Check sheet for the drawn part. Datum: minimum x, y, z corner. Units: mm. Round coordinates to 2 decimals unless told otherwise and drop trailing zeros. Write each loop counter-clockwise with the first axis right and the second up, starting at its lowest first coordinate (ties: lowest second). Pieces come first, ordered by that corner, then holes. Notation, with made-up numbers: (-7, -12) - (31, -12) arc R11 ccw to (31, 8) - close; hole circle Ø5 at (13, -37.5). An arc over 180 degrees is marked (long way). Return JSON: item names as keys, results as strings. Group by question number.
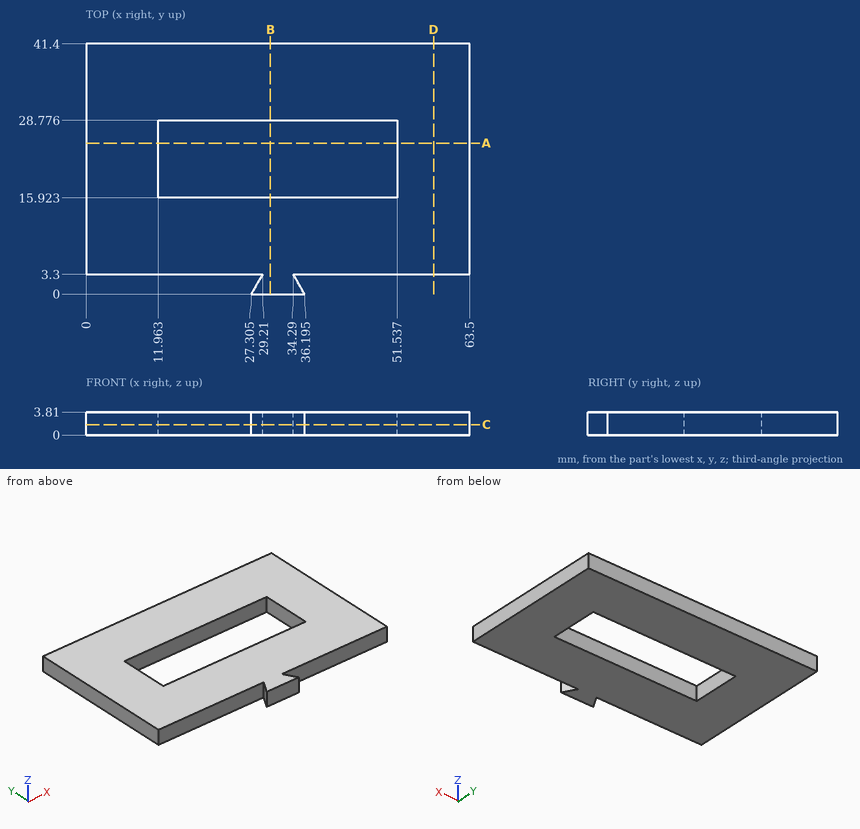
1. Depth check by flat-ended pin: pin 1 Ø1.5 at (x, z) = (18, 2.5) entering from -Y; pin 2 Ø6 at (x, y) = (29.5, 20.5) entering from -Z. Enter the tip coordinate at first touch or a pass-through.
2. Section check C-C (z = 1.75). Enter the section's corners in (x, y) (1 decimal), and give its area (3 significant figures).
3. Section check D-D (x = 57.5). Enter the section's corners in (y, z), and give its area (3 significant figures).
4. Material ranges on line 1 along X through (y, z) = (19.5, 1.3); line 2 along Y through (x, z) = (41, 3.2) (1 decimal); line 3 along Y through (x, z) = (58.5, 1.75), recorded low to high.
5. Section check A-A (y = 25). Enter the section's corners in (x, z).
6. Section check B-B (x = 30.5). Enter the section's corners in (y, z) (1 decimal), and give its area (3 significant figures).
Result sheet:
{
 "1": {"pin 1": "stops at y = 3.3", "pin 2": "passes through"},
 "2": {"outline": "(0, 3.3) - (29.2, 3.3) - (27.3, 0) - (36.2, 0) - (34.3, 3.3) - (63.5, 3.3) - (63.5, 41.4) - (0, 41.4) - close; hole (12, 15.9) - (51.5, 15.9) - (51.5, 28.8) - (12, 28.8) - close", "area": "1,930 mm²"},
 "3": {"outline": "(3.3, 0) - (41.4, 0) - (41.4, 3.81) - (3.3, 3.81) - close", "area": "145 mm²"},
 "4": {"line 1": "x = 0 to 11.96, 51.54 to 63.5", "line 2": "y = 3.3 to 15.9, 28.8 to 41.4", "line 3": "y = 3.3 to 41.4"},
 "5": {"outline": "(0, 0) - (11.96, 0) - (11.96, 3.81) - (0, 3.81) - close; (51.54, 0) - (63.5, 0) - (63.5, 3.81) - (51.54, 3.81) - close"},
 "6": {"outline": "(0, 0) - (15.9, 0) - (15.9, 3.8) - (0, 3.8) - close; (28.8, 0) - (41.4, 0) - (41.4, 3.8) - (28.8, 3.8) - close", "area": "109 mm²"}
}
